Input: dimensioned drawing with shaded views. Units: mm. Origin: part minimum x, y, z. A direction names the side the tool comes from. Round coordinates to 2 decimals unless told otherwise and drop trailing zeros. Loops run counter-clockwise (first coordinate to the right, second up) from the corner with the lowest first, then second, coordinate; pieces in that order, holes last. Notation, with made-up numbers: (64, 56) - (76, 56) arc R10 cw to (76, 68) - close; hole circle Ø6 at (26, 10). An arc over 180 degrees is marked (long way). One line per question, with ' | ' between items. Start each with the question number.
Item 1: First-contact query: pin 1 (1.8 mm diameter, centred on x = 20.701, z = 3.175, fed in from -Y); pin 2 (5 mm diameter, centred on y = 10.5, z = 15, fed in from +X) (3 decimals); pin 3 (1.7 mm diameter, centred on y = 10, z = 11.5, fed in from -X) (3 decimals); pin 4 (1 mm diameter, centred on x = 28, z = 12, fed in from +Y). Flat tips, straight axial feed; report the tip coordinate or a pass-through.
Item 2: Section D-D, the plane y = 5.25. Give the number of separate pieces and of enclosed holes in the cut face, plus the area to 3 significant figures.
Item 3: Set-up query: the marked faces 1, 2, 3 and 4. Return all of +Z, -Z, +X, -X, +Y, -Y with unobstructed straight access to the full face (end or side cutting, diameter ignored); none if empty.
Item 4: Material intervals for line 1 along X through (y, z) = (8.5, 12.5) (3 decimals); line 2 along Y through (x, z) = (24, 13.5) (1 decimal); line 3 along X through (y, z) = (14.25, 4), sorted ascending.
Item 5: Section C-C, the plane y = 10. Return loops of the section in (x, z) (3 decimals).
Item 6: Draft query along X for the marked faces 5, 6 and 7. Return one class per face: pulls with the +X half, pulls with the -X half, needs draft (parallel to the pull), parting line crosses it, or undercut.
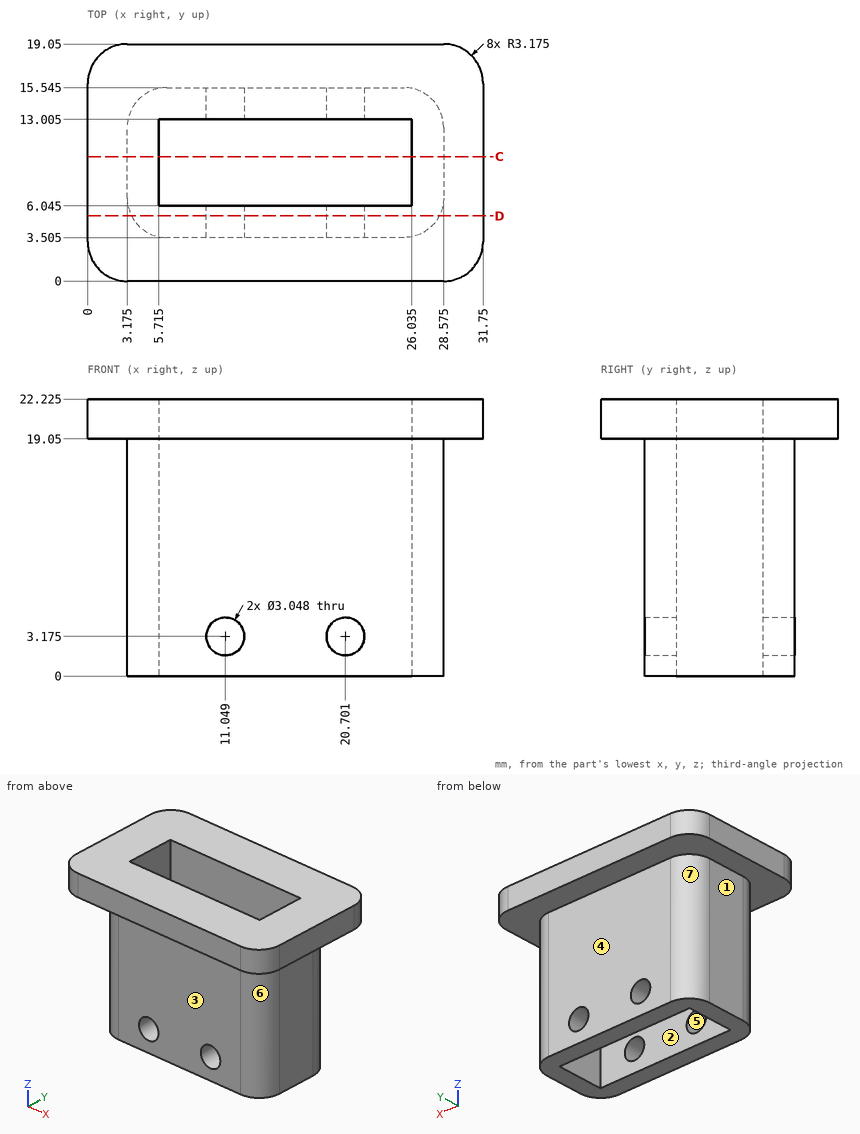
Return value:
1) pin 1: through | pin 2: x = 28.575 | pin 3: x = 3.175 | pin 4: y = 14.75
2) separate pieces: 1 | enclosed holes: 2 | area: 557 mm2
3) face 1: -Z, -X, +Y, -Y | face 2: +Z, -Z | face 3: -Z, +X, -X, -Y | face 4: -Z, +X, -X, +Y
4) line 1: 3.175 to 5.715, 26.035 to 28.575 | line 2: 3.5 to 6, 13 to 15.5 | line 3: 3.79 to 9.77, 12.33 to 19.42, 21.98 to 27.96
5) outline: (0, 19.05) - (3.175, 19.05) - (3.175, 0) - (5.715, 0) - (5.715, 22.225) - (0, 22.225) - close; (26.035, 0) - (28.575, 0) - (28.575, 19.05) - (31.75, 19.05) - (31.75, 22.225) - (26.035, 22.225) - close
6) face 5: undercut | face 6: pulls with the +X half | face 7: pulls with the -X half
